```python
from build123d import *

# Parameters (mm, degrees)
F1_DEPTH = 25


with BuildPart() as f1:
    # F0 (on Top) → F1 (new body)
    with BuildSketch(Plane.XY):
        with BuildLine():
            Line((-160.09872, 248.367966), (-172.318979, 248.367966))
            Line((-172.318979, 248.367966), (-172.318979, 48.367966))
            Line((-172.318979, 48.367966), (37.681021, 48.367966))
            Line((37.681021, 48.367966), (37.681021, 59.875305))
            ThreePointArc((37.681021, 59.875305), (33.991015, 69.728429), (24.736483, 74.733807))
            ThreePointArc((24.736483, 74.733807), (-86.259099, 128.13192), (-145.367485, 236.194754))
            ThreePointArc((-145.367485, 236.194754), (-150.543664, 244.930877), (-160.09872, 248.367966))
        make_face()
    extrude(amount=F1_DEPTH)


solid = f1.part
```
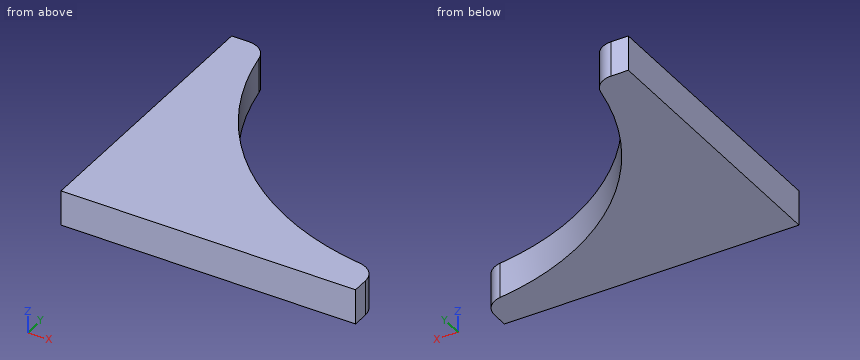
Design review of the part built by this model. Coordinates are the model's own, in mm. Round coordinates to 2 decimals unless told otherwise and drop trailing zeros. Write each loop counter-clockwise with the first axis right and the second up, starting at its lowest first coordinate (ties: lowest second). Pieces come first, ordered by that corner, then holes.
Item 1: We need section B-B on x = 1. Write out the cut boundary in (y, z).
Item 2: Clearance check with flat-ended pins moving along their axes: pin 1 Ø1.5 at (x, z) = (-1.5, 17.5) entering from +Y; pin 2 Ø1.5 at (x, z) = (-41.5, 5.5) entering from +Y; pin 3 Ø10 at (x, z) = (1, 17.5) entering from +Y. State where each tip first meets the part, or that it passes through.
Item 3: For probe 1 along X at (y, z) = (214, 10); probe 2 along X at (y, z) = (102, 11); probe 3 along Y at (x, z) = (-93.5, 23.25), list the stretches that pass through material, from the lowest coordinate up.
Item 4: We need section C-C on y = 91. Write out the cut boundary in (x, z).
Item 5: We need section A-A on z = 21.5. Write out the cut boundary in (x, y).
Returned:
1. outline: (48.37, 0) - (79.49, 0) - (79.49, 25) - (48.37, 25) - close
2. pin 1: stops at y = 80.37
2. pin 2: stops at y = 96.43
2. pin 3: stops at y = 80.87
3. probe 1: x = -172.32 to -139.78
3. probe 2: x = -172.32 to -52.04
3. probe 3: y = 48.37 to 135.36
4. outline: (-172.32, 0) - (-31.24, 0) - (-31.24, 25) - (-172.32, 25) - close
5. outline: (-172.32, 48.37) - (37.68, 48.37) - (37.68, 59.88) arc R15 ccw to (24.74, 74.73) arc R201.29 cw to (-145.37, 236.19) arc R15 ccw to (-160.1, 248.37) - (-172.32, 248.37) - close
